```python
from build123d import *

# Parameters (mm, degrees)
F0_W     = 63.5
F0_H     = 38.1
F1_DEPTH = 127
F3_W     = 6.35
F3_H     = 6.35
F4_DEPTH = 127
F2_W     = 6.35
F2_H     = 6.35
F5_DEPTH = 127


with BuildPart() as f1:
    # F0 (on Front) → F1 (new body)
    with BuildSketch(Plane.XZ):
        Rectangle(F0_W, F0_H)
    extrude(amount=F1_DEPTH)

    # F3 (on Front) → F4 (cut)
    with BuildSketch(Plane.XZ):
        with Locations((-28.984677, 16.079839)):
            Rectangle(F3_W, F3_H)
    extrude(amount=F4_DEPTH, mode=Mode.SUBTRACT)

    # F2 (on Front) → F5 (cut)
    with BuildSketch(Plane.XZ):
        with Locations((28.718387, 15.997903)):
            Rectangle(F2_W, F2_H)
    extrude(amount=F5_DEPTH, mode=Mode.SUBTRACT)


solid = f1.part
```
Source: CAD feature listing. Evaluate the final solid. Frame: model axes, mm. A direction names the side the tool comes from. Give positions to 0.01 mm unless a question says otherwise; leave off trailing zeros. Write each loop counter-clockwise with the first axis right and the second up, starting at its lowest first coordinate (ties: lowest second). Pieces come first, ordered by that corner, then holes.
1. Section query B-B (x = 27.5). Return the cut outline in (y, z).
2. Access query for faces 1 (the face through (0, 0, 0)), 2 (the face through (-29, -63, 12.905)), 3 (the face through (25.543, -63, 16)). Directions: +Z, -Z, +X, -X, +Y, -Y. A direction counts if a zero-diameter tool reaches every point of the face in a straight line with its end or side. Return the directions, or none.
3. Material intervals for line 1 along X through (y, z) = (-21.5, 13), sorted ascending.
4. First-contact query: pin 1 (6.5 mm diameter, centred on x = -30, y = -36.5, fed in from +Z); pin 2 (3 mm diameter, centred on x = 30, y = -60, fed in from +Z); pin 3 (1.9 mm diameter, centred on y = -57, z = 17, fed in from +X). Flat tips, straight axial feed; report the tip coordinate or a pass-through.
5. Section query A-A (y = -61). Return the cut outline in (x, z), then the cut area to 3 significant figures.
Output values:
1. outline: (-127, -19.05) - (0, -19.05) - (0, 12.82) - (-127, 12.82) - close
2. face 1: +Z, -Z, +X, -X, +Y
2. face 2: +Z, -X, +Y, -Y
2. face 3: +Z, +X, +Y, -Y
3. line 1: x = -25.81 to 25.54
4. pin 1: stops at z = 12.9
4. pin 2: stops at z = 12.82
4. pin 3: stops at x = 25.54
5. outline: (-31.75, -19.05) - (31.75, -19.05) - (31.75, 12.82) - (25.54, 12.82) - (25.54, 19.05) - (-25.81, 19.05) - (-25.81, 12.9) - (-31.75, 12.9) - close
5. area: 2,340 mm2
